Input: part model. Units: mm. Frame: model coordinates. A direction names the side the tool comes from. Coordinates: 2 decimals unless noted, no trailing zeros. Order: outer loops, then holes, each group sorted by start corner. A loop starts at its lowest first (then second) coordinate and runs counter-clockwise, first axis right, second up.
from build123d import *

# Parameters (mm, degrees)
SKETCH1_R           = 1.5
BOSS_EXTRUDE1_DEPTH = 3.175
FILLET1_R           = 5


with BuildPart() as part:
    # Sketch1 → Boss-Extrude1 (new body)
    with BuildSketch(Plane.XY):
        Polygon((0, 37.5), (0, 0), (25, 0), (25, 75), (-15, 75), (-15, 37.5), align=None)
        with Locations((12.5, 6)):
            Circle(SKETCH1_R, mode=Mode.SUBTRACT)
        with Locations((12.5, 37.5)):
            Circle(SKETCH1_R, mode=Mode.SUBTRACT)
        with Locations((12.5, 69)):
            Circle(SKETCH1_R, mode=Mode.SUBTRACT)
    extrude(amount=BOSS_EXTRUDE1_DEPTH)

    # Fillet1
    fillet1_edges = [part.edges().sort_by_distance(p)[0] for p in [
        (25, 75, 1.5875),
        (25, 0, 1.5875),
        (0, 0, 1.5875),
        (0, 37.5, 1.5875),
        (-15, 37.5, 1.5875),
        (-15, 75, 1.5875),
    ]]
    fillet(fillet1_edges, radius=FILLET1_R)


solid = part.part
Item 1: Cut plane D-D on y = 6. Return loops of the section in (x, z) (3 decimals), then the cut area to 4 significant figures.
Response values:
outline: (0, 0) - (11, 0) - (11, 3.175) - (0, 3.175) - close; (14, 0) - (25, 0) - (25, 3.175) - (14, 3.175) - close
area: 69.85 mm2
Item 2: Pin query (flat end, axial travel): pin 1 Ø1.8 at (x, y) = (12.5, 37.5) entering from +Z; pin 2 Ø1.6 at (y, z) = (25.5, 1) entering from -X; pin 3 Ø4 at (x, y) = (12.5, 6) entering from -Z; pin 4 Ø1 at (x, z) = (-8.5, 1.5) entering from -Y. Return the tip coordinate at first contact, or that it passes through.
Response values:
pin 1: passes through
pin 2: stops at x = 0
pin 3: stops at z = 0
pin 4: stops at y = 37.5
Item 3: Cut plane B-B on y = 69. Return loops of the section in (x, z) (3 decimals), then the cut area to 3 significant figures.
Response values:
outline: (-15, 0) - (11, 0) - (11, 3.175) - (-15, 3.175) - close; (14, 0) - (25, 0) - (25, 3.175) - (14, 3.175) - close
area: 117 mm2
Item 4: Access query for faces 5 (the face through (9, 38, 0)), 6 (the face through (0, 19, 2)). Directions: +Z, -Z, +X, -X, +Y, -Y. A direction counts if a zero-diameter tool reaches every point of the face in a straight line with its end or side. Return the directions, or none.
Response values:
face 5: -Z, +X, -X, +Y, -Y
face 6: +Z, -Z, -X, -Y
Item 5: Cut plane A-A on x = 12.5. Return loops of the section in (y, z) (3 decimals), then the cut area to 3 significant figures.
Response values:
outline: (0, 0) - (4.5, 0) - (4.5, 3.175) - (0, 3.175) - close; (7.5, 0) - (36, 0) - (36, 3.175) - (7.5, 3.175) - close; (39, 0) - (67.5, 0) - (67.5, 3.175) - (39, 3.175) - close; (70.5, 0) - (75, 0) - (75, 3.175) - (70.5, 3.175) - close
area: 210 mm2
Item 6: Ray query, probe 1 along Y at (x, z) = (12.5, 2); probe 2 along X at (y, z) = (69, 1.25); probe 3 along Y at (x, z) = (-10, 0.45). Return the intervals inside material, ascending.
Response values:
probe 1: y = 0 to 4.5, 7.5 to 36, 39 to 67.5, 70.5 to 75
probe 2: x = -15 to 11, 14 to 25
probe 3: y = 37.5 to 75
Item 7: Cut plane C-C on z = 1. Return loops of the section in (x, y).
Response values:
outline: (-15, 42.5) arc R5 ccw to (-10, 37.5) - (-5, 37.5) arc R5 cw to (0, 32.5) - (0, 5) arc R5 ccw to (5, 0) - (20, 0) arc R5 ccw to (25, 5) - (25, 70) arc R5 ccw to (20, 75) - (-10, 75) arc R5 ccw to (-15, 70) - close; hole circle Ø3 at (12.5, 6); hole circle Ø3 at (12.5, 37.5); hole circle Ø3 at (12.5, 69)
Item 8: Draft query along X for faces 1 (the face through (1, 2, 2)), 2 (the face through (13.306, 70.265, 1.565)), 3 (the face through (25, 37, 2)), 4 (the face through (12, 0, 2)). Return one class per face: pulls with the +X half, pulls with the -X half, needs draft (parallel to the pull), parting line crosses it, or undercut.
Response values:
face 1: pulls with the -X half
face 2: undercut
face 3: pulls with the +X half
face 4: needs draft
